from build123d import *

# Parameters (mm, degrees)
F0_R     = 3
F1_DEPTH = 3


with BuildPart() as f1:
    # F0 (on Top) → F1 (new body)
    with BuildSketch(Plane.XY):
        with BuildLine():
            ThreePointArc((2.243782, 25.522082), (2.11952, 25.894266), (1.999187, 26.267739))
            ThreePointArc((1.999187, 26.267739), (2.097618, 25.887082), (2.243782, 25.522082))
        make_face()
        with BuildLine():
            ThreePointArc((45.522983, 73.860736), (45.144109, 73.965821), (44.754928, 74.021739))
            ThreePointArc((44.754928, 74.021739), (45.13938, 73.943261), (45.522983, 73.860736))
        make_face()
        with BuildLine():
            ThreePointArc((65.50129, 12.956179), (65.2411, 12.662473), (64.97783, 12.371525))
            ThreePointArc((64.97783, 12.371525), (65.258273, 12.647097), (65.50129, 12.956179))
        make_face()
        with BuildLine():
            ThreePointArc((32.085906, 68.314754), (33.728593, 71.692394), (30.881851, 74.142482))
            ThreePointArc((30.881851, 74.142482), (5.617411, 56.734654), (1.999187, 26.267739))
            ThreePointArc((1.999187, 26.267739), (2.11952, 25.894266), (2.243782, 25.522082))
            ThreePointArc((2.243782, 25.522082), (5.767854, 23.860831), (8.095696, 26.984929))
            ThreePointArc((8.095696, 26.984929), (30.811472, 33.520681), (13.520687, 17.40388))
            ThreePointArc((13.520687, 17.40388), (9.774222, 17.137669), (9.075754, 13.447274))
            ThreePointArc((9.075754, 13.447274), (36.783596, 0.271541), (64.97783, 12.371525))
            ThreePointArc((64.97783, 12.371525), (65.2411, 12.662473), (65.50129, 12.956179))
            ThreePointArc((65.50129, 12.956179), (65.17794, 16.83874), (61.30847, 17.292661))
            ThreePointArc((61.30847, 17.292661), (44.290455, 33.697224), (66.893407, 26.781366))
            ThreePointArc((66.893407, 26.781366), (68.997185, 23.669938), (72.542395, 24.910244))
            ThreePointArc((72.542395, 24.910244), (70.098993, 55.493805), (45.522983, 73.860736))
            ThreePointArc((45.522983, 73.860736), (45.13938, 73.943261), (44.754928, 74.021739))
            ThreePointArc((44.754928, 74.021739), (41.554206, 71.800429), (43.095833, 68.22241))
            ThreePointArc((43.095833, 68.22241), (37.398073, 45.282094), (32.085906, 68.314754))
        make_face()
        with Locations((37.5, 37.5)):
            Circle(F0_R, mode=Mode.SUBTRACT)
    extrude(amount=F1_DEPTH)


solid = f1.part
Geometry check sheet. Reference: the model listing, model coordinates, mm. A direction names the side the tool comes from. Round coordinates to 2 decimals unless told otherwise and drop trailing zeros. Write each loop counter-clockwise with the first axis right and the second up, starting at its lowest first coordinate (ties: lowest second). Pieces come first, ordered by that corner, then holes.
Item 1: Material ranges on line 1 along X through (y, z) = (38, 0.3); line 2 along Y through (x, z) = (37.5, 1.15); line 3 along X through (y, z) = (25, 0.2), recorded low to high.
Determined:
line 1: x = 0.27 to 14.06, 26.41 to 34.54, 40.46 to 48.59, 60.94 to 74.73
line 2: y = 0.26 to 34.5, 40.5 to 45.28
line 3: x = 2.56 to 7.48, 32.12 to 42.88, 67.33 to 72.57
Item 2: Access from +Z, -Z, +X, -X, +Y, -Y to the whole of each face (thin tool, end or side, straight path). Record for faces 1 (the face through (45, 38, 0)), 2 (the face through (41.57, 71.86, 1.48)).
Determined:
face 1: -Z, +X, -X, +Y, -Y
face 2: +Z, -Z
Item 3: Section check B-B (y = 37.5). Record the boundary of the cut face in (x, z).
Determined:
outline: (0.26, 0) - (13.28, 0) - (13.28, 3) - (0.26, 3) - close; (27.19, 0) - (34.5, 0) - (34.5, 3) - (27.19, 3) - close; (40.5, 0) - (47.81, 0) - (47.81, 3) - (40.5, 3) - close; (61.72, 0) - (74.74, 0) - (74.74, 3) - (61.72, 3) - close
Item 4: Mould release check, pull along X, two halves, no side actions. Record for faces 3 (the face through (70.311, 55.105, 1.479)), 4 (the face through (33.74, 71.64, 1.48)), 5 (the face through (45, 38, 3)): +X half, -X half, draft (parallel to the pull), parting line (faces both ways), or undercut.
Determined:
face 3: +X half
face 4: undercut
face 5: draft
Item 5: Go/stop test with flat-tipped pins: pin 1 Ø1.5 at (y, z) = (55.5, 0.5) entering from -X; pin 2 Ø8 at (x, y) = (31, 64) entering from +Z. Record where each tip stops, or that it passes through.
Determined:
pin 1: stops at x = 4.5
pin 2: stops at z = 3
Item 6: Section check C-C (y = 61). Record the boundary of the cut face in (x, z).
Determined:
outline: (8.62, 0) - (25.88, 0) - (25.88, 3) - (8.62, 3) - close; (49.12, 0) - (66.38, 0) - (66.38, 3) - (49.12, 3) - close
Item 7: Section check A-A (x = 37.5). Record the boundary of the cut face in (y, z), plus the area to 3 significant figures.
Determined:
outline: (0.26, 0) - (34.5, 0) - (34.5, 3) - (0.26, 3) - close; (40.5, 0) - (45.28, 0) - (45.28, 3) - (40.5, 3) - close
area: 117 mm2
Item 8: Section check D-D (z = 0.8). Record the boundary of the cut face in (x, y) (1 decimal), plus the area to 3 significant figures.
Determined:
outline: (2, 26.3) arc R3.1 ccw to (2.2, 25.5) arc R3.1 ccw to (8.1, 27) arc R12.2 cw (long way) to (13.5, 17.4) arc R3.1 ccw to (9.1, 13.4) arc R37.2 ccw to (65, 12.4) arc R3.1 ccw to (65.5, 13) arc R3.1 ccw to (61.3, 17.3) arc R12.2 cw (long way) to (66.9, 26.8) arc R3.1 ccw to (72.5, 24.9) arc R37.2 ccw to (45.5, 73.9) arc R3.1 ccw to (44.8, 74) arc R3.1 ccw to (43.1, 68.2) arc R12.2 cw (long way) to (32.1, 68.3) arc R3.1 ccw to (30.9, 74.1) arc R37.2 ccw to start; hole circle Ø6 at (37.5, 37.5)
area: 2,790 mm2
